Can you work these out from the model? Positions are in its coordinate system, mm. A direction names the side the tool comes from. Coordinates: 2 decimals unless noted, no trailing zeros. Loops run counter-clockwise (first coordinate to the right, second up) from the corner with the lowest first, then second, coordinate; pieces in that order, holes last.
```python
from build123d import *

# Parameters (mm, degrees)
SKETCH1_R           = 8
BOSS_EXTRUDE1_DEPTH = 5
SKETCH2_W           = 6.4
SKETCH2_H           = 3.2
CUT_EXTRUDE1_DEPTH  = 2


with BuildPart() as part:
    # Sketch1 → Boss-Extrude1 (new body)
    with BuildSketch(Plane(origin=(0, 0, 0), x_dir=(1, 0, 0), z_dir=(0, 1, 0))):
        with Locations(Location((0, 0, 0), (0, 0, 270))):
            Circle(SKETCH1_R)
    extrude(amount=BOSS_EXTRUDE1_DEPTH)

    # Sketch2 → Cut-Extrude1 (cut)
    with BuildSketch(Plane.XZ):
        Rectangle(SKETCH2_W, SKETCH2_H)
    extrude(amount=-CUT_EXTRUDE1_DEPTH, mode=Mode.SUBTRACT)

    # Sketch3 → Cut-Revolve1 (revolve, cut)
    with BuildSketch(Plane.XY, mode=Mode.PRIVATE) as cut_revolve1_sk:
        Polygon((0, 3), (-3.4, 3), (-3.4, 4), (-5.25, 4), (-5.25, 5), (0, 5), align=None)
    revolve(cut_revolve1_sk.sketch.rotate(Axis((0, 0, 0), (0, -1, 0)), 270), axis=Axis((0, 0, 0), (0, -1, 0)), mode=Mode.SUBTRACT)


solid = part.part
```
Item 1: We'd pull the mould along X, two halves only. Please class faces 1 (the face through (3.4, 4, -1.1)), 2 (the face through (0, 0, 2)), 3 (the face through (-7.81, 2.46, -1.73)): +X half, -X half, draft (parallel to the pull), parting line (faces both ways), or undercut.
Results are:
face 1: undercut
face 2: draft
face 3: parting line
Item 2: I need wall thicknesses on line 1 along X through (y, z) = (3.65, 0); line 2 along X through (y, z) = (4.7, 0); line 3 along Y through (x, z) = (1, -4.5). Which ranges of each line are inside material? Lowest first, please.
Results are:
line 1: x = -8 to -3.4, 3.4 to 8
line 2: x = -8 to -5.25, 5.25 to 8
line 3: y = 0 to 4
Item 3: On a 3-axis mill with a long thin cutter (end or side, diameter ignored), from which of +Z, -Z, +X, -X, +Y, -Y can I reach the whole of each face in a straight line? I mean faces 4 (the face through (-1.7, 5, 5.2)), 5 (the face through (3.32, 3.51, -0.74)), 6 (the face through (3.2, 1, 0)). Say none if no direction works.
Results are:
face 4: +Z, -Z, +X, -X, +Y
face 5: +Y
face 6: -Y
Item 4: Suppose I cut it at B-B, the plane x = 0. Please give me the cut outline in (y, z), plus the area to 3 significant figures.
Results are:
outline: (0, -8) - (5, -8) - (5, -5.25) - (4, -5.25) - (4, -3.4) - (3, -3.4) - (3, 3.4) - (4, 3.4) - (4, 5.25) - (5, 5.25) - (5, 8) - (0, 8) - (0, 1.6) - (2, 1.6) - (2, -1.6) - (0, -1.6) - close
area: 56.3 mm2
Item 5: Suppose I cut it at D-D, the plane z = -3. Please give me the cut outline in (x, y).
Results are:
outline: (-7.42, 0) - (7.42, 0) - (7.42, 5) - (4.31, 5) - (4.31, 4) - (1.6, 4) - (1.6, 3) - (-1.6, 3) - (-1.6, 4) - (-4.31, 4) - (-4.31, 5) - (-7.42, 5) - close
Item 6: Suppose I cut it at A-A, the plane z = 0. Please give me the cut outline in (x, y), plus the area to 3 significant figures.
Results are:
outline: (-8, 0) - (-3.2, 0) - (-3.2, 2) - (3.2, 2) - (3.2, 0) - (8, 0) - (8, 5) - (5.25, 5) - (5.25, 4) - (3.4, 4) - (3.4, 3) - (-3.4, 3) - (-3.4, 4) - (-5.25, 4) - (-5.25, 5) - (-8, 5) - close
area: 49.9 mm2
Item 7: Suppose I cut it at C-C, the plane y = 1.8. Please give me the cut outline in (x, z), plus the area to 3 significant figures.
Results are:
outline: circle Ø16 at (0, 0); hole (-3.2, -1.6) - (3.2, -1.6) - (3.2, 1.6) - (-3.2, 1.6) - close
area: 181 mm2
Item 8: I'm going to push flat-ended pins straight in: P1, Ø5.5, axis at x = 1, z = 1, coming from the +Y side; P2, Ø1.5, axis at y = 2.5, z = 6, coming from the +X side; P3, Ø2, axis at y = 4, z = 1.5, coming from the +X side. Where does each tip first touch, or does it pass through?
Results are:
P1: stops at y = 4
P2: stops at x = 6.04
P3: stops at x = 7.98
